Geometry check sheet. Reference: the model listing, model coordinates, mm. Face numbers are marked on the shaded views. A direction names the side the tool comes from. Coordinates: 2 decimals unless noted, no trailing zeros. Write each loop counter-clockwise with the first axis right and the second up, starting at its lowest first coordinate (ties: lowest second). Pieces come first, ordered by that corner, then holes. Notation, with made-up numbers: (-28.75, 14) - (28.25, 14) arc R21 cw to (28.25, 41) - close; hole circle Ø10 at (7.25, 36). An arc over 180 degrees is marked (long way). Answer as a JSON object with one key per item and string values. Group by question number.
from build123d import *

# Parameters (mm, degrees)
SKETCH1_R           = 1.5
BOSS_EXTRUDE1_DEPTH = 3
SKETCH2_W           = 1.19
SKETCH2_H           = 4.79
CUT_EXTRUDE1_DEPTH  = 10


with BuildPart() as part:
    # Sketch1 → Boss-Extrude1 (new body)
    with BuildSketch(Plane.XY):
        with BuildLine():
            Line((20.555, 4.79), (20.555, 0))
            Line((20.555, 0), (0, 0))
            Line((0, 0), (0, 4.79))
            Line((0, 4.79), (16.23, 4.79))
            ThreePointArc((16.23, 4.79), (17.627100654, 8.162899346), (21, 9.56))
            Line((21, 9.56), (21, 4.79))
            Line((21, 4.79), (20.555, 4.79))
        make_face()
        with Locations((3, 2.5)):
            Circle(SKETCH1_R, mode=Mode.SUBTRACT)
        with Locations((16.23, 2.5)):
            Circle(SKETCH1_R, mode=Mode.SUBTRACT)
    boss_extrude1 = extrude(amount=BOSS_EXTRUDE1_DEPTH)

    # Mirror1: Boss-Extrude1 across plane
    add(boss_extrude1.mirror(Plane(origin=(21, 9.56, 3), x_dir=(0, 0, 1), z_dir=(-1, 0, 0))))

    # Sketch2 → Cut-Extrude1 (cut)
    with BuildSketch(Plane.XY.offset(3)):
        with Locations((21.15, 2.395)):
            Rectangle(SKETCH2_W, SKETCH2_H)
    extrude(amount=-CUT_EXTRUDE1_DEPTH, mode=Mode.SUBTRACT)


solid = part.part
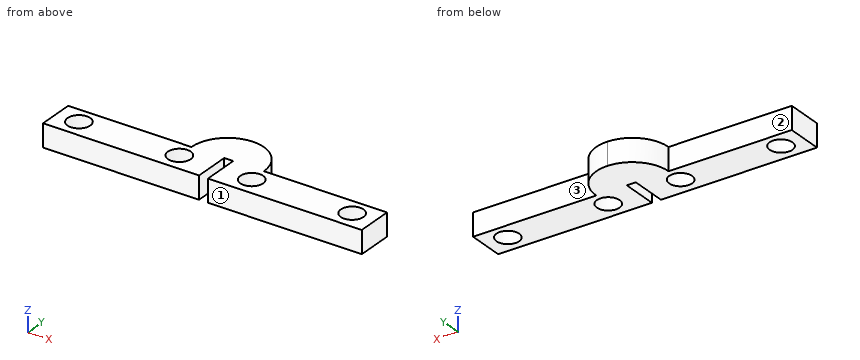
(1) Material ranges on L1, parallel to Y at x = 39, z = 2.3; L2, parallel to X at y = 4.5, z = 0.6 (3 decimals); L3, parallel to X at y = 3.75, z = 2.6 (3 decimals), recorded low to high. Write a range as [from, to].
(2) Set-up check for the marked faces 1, 2 and 3: record each of +Z, -Z, +X, -X, +Y, -Y from which the full face is reachable in a straight line by a thin tool's end or side.
(3) Section check B-B (y = 2.5). Record the cut outline in (x, z) (3 decimals), and give its area (3 significant figures).
(4) Gauge pin test, flat end, axial feed: pin 1 (2.5 mm diameter, centred on x = 16.23, y = 2.5, fed in from -Z). Record the tip position at first contact, or that the pin passes through.
(5) Section check A-A (x = 3). Record the cut outline in (y, z), and give its area (3 significant figures).
(6) Section check C-C (z = 1.5). Record the cut outline in (x, y) (3 decimals), and give its area (3 significant figures).
(7) Section check D-D (x = 12). Record the cut outline in (y, z), and give its area (3 significant figures).
Conclusion:
{
 "1": {"L1": "y = [0, 1], [4, 4.79]", "L2": "x = [0, 20.555], [21.745, 42]", "L3": "x = [0, 2.171], [3.829, 15.401], [17.059, 20.555], [21.745, 24.941], [26.599, 38.171], [39.829, 42]"},
 "2": {"face 1": "+Z, -Z, +X, -X, -Y", "face 2": "+Z, -Z, -X, +Y", "face 3": "+Z, -Z, +X, +Y"},
 "3": {"outline": "(0, 0) - (1.5, 0) - (1.5, 3) - (0, 3) - close; (4.5, 0) - (14.73, 0) - (14.73, 3) - (4.5, 3) - close; (17.73, 0) - (20.555, 0) - (20.555, 3) - (17.73, 3) - close; (21.745, 0) - (24.27, 0) - (24.27, 3) - (21.745, 3) - close; (27.27, 0) - (37.5, 0) - (37.5, 3) - (27.27, 3) - close; (40.5, 0) - (42, 0) - (42, 3) - (40.5, 3) - close", "area": "86.4 mm^2"},
 "4": {"pin 1": "passes through"},
 "5": {"outline": "(0, 0) - (1, 0) - (1, 3) - (0, 3) - close; (4, 0) - (4.79, 0) - (4.79, 3) - (4, 3) - close", "area": "5.37 mm^2"},
 "6": {"outline": "(0, 0) - (20.555, 0) - (20.555, 4.79) - (21.745, 4.79) - (21.745, 0) - (42, 0) - (42, 4.79) - (25.77, 4.79) arc R4.77 ccw to (16.23, 4.79) - (0, 4.79) - close; hole circle Ø3 at (3, 2.5); hole circle Ø3 at (16.23, 2.5); hole circle Ø3 at (25.77, 2.5); hole circle Ø3 at (39, 2.5)", "area": "203 mm^2"},
 "7": {"outline": "(0, 0) - (4.79, 0) - (4.79, 3) - (0, 3) - close", "area": "14.4 mm^2"}
}
